from build123d import *

# Parameters (mm, degrees)
SKETCH1_R                = 30
SKETCH1_R_2              = 25
BOSS_EXTRUDE1_DEPTH      = 5
SKETCH2_R                = 25
BOSS_EXTRUDE2_DEPTH      = 2
CUT_EXTRUDE1_DEPTH       = 43.720018727
CUT_EXTRUDE1_DEPTH_BACK  = 43.720018727
SKETCH2_4_R              = 5
BOSS_EXTRUDE3_DEPTH      = 3
BOSS_EXTRUDE3_DEPTH_BACK = 7
SKETCH3_R                = 5
SKETCH3_R_2              = 2
CUT_EXTRUDE2_DEPTH       = 44
CUT_EXTRUDE2_DEPTH_BACK  = 44
SKETCH4_R                = 5
CHAMFER1_SIZE            = 0.5


with BuildPart() as part:
    # Sketch1 → Boss-Extrude1 (new, symmetric)
    with BuildSketch(Plane.XY):
        Circle(SKETCH1_R)
        Circle(SKETCH1_R_2, mode=Mode.SUBTRACT)
    extrude(amount=BOSS_EXTRUDE1_DEPTH, both=True)

    # Sketch2 → Boss-Extrude2 (add, symmetric)
    with BuildSketch(Plane.XY):
        Circle(SKETCH2_R)
    extrude(amount=BOSS_EXTRUDE2_DEPTH, both=True)

    # Sketch2_4 → Cut-Extrude1 (cut, two sides: drawn at the far end of the back side and taken through both)
    with BuildSketch(Plane.XY.offset(-CUT_EXTRUDE1_DEPTH_BACK)):
        Circle(SKETCH2_4_R)
    extrude(amount=CUT_EXTRUDE1_DEPTH + CUT_EXTRUDE1_DEPTH_BACK, mode=Mode.SUBTRACT)

    # Sketch3 → Boss-Extrude3 (add, two sides: drawn at the far end of the back side and taken through both)
    with BuildSketch(Plane(origin=(0, 0, -2), x_dir=(-1, 0, 0), z_dir=(0, 0, -1)).offset(-BOSS_EXTRUDE3_DEPTH_BACK)):
        Circle(SKETCH3_R)
        Circle(SKETCH3_R_2, mode=Mode.SUBTRACT)
    extrude(amount=BOSS_EXTRUDE3_DEPTH + BOSS_EXTRUDE3_DEPTH_BACK)

    # Sketch4 → Cut-Extrude2 (cut, two sides: drawn at the far end of the back side and taken through both)
    with BuildSketch(Plane(origin=(0, 0, -2), x_dir=(-1, 0, 0), z_dir=(0, 0, -1)).offset(-CUT_EXTRUDE2_DEPTH_BACK)):
        with Locations(Location((0, 18, 0), (0, 0, 180))):
            Circle(SKETCH4_R)
        with Locations(Location((12.727922061, 12.727922061, 0), (0, 0, 180))):
            Circle(SKETCH4_R)
        with Locations(Location((18, 0, 0), (0, 0, 180))):
            Circle(SKETCH4_R)
        with Locations(Location((12.727922061, -12.727922061, 0), (0, 0, 180))):
            Circle(SKETCH4_R)
        with Locations(Location((0, -18, 0), (0, 0, 180))):
            Circle(SKETCH4_R)
        with Locations(Location((-12.727922061, -12.727922061, 0), (0, 0, 180))):
            Circle(SKETCH4_R)
        with Locations(Location((-18, 0, 0), (0, 0, 180))):
            Circle(SKETCH4_R)
        with Locations(Location((-12.727922061, 12.727922061, 0), (0, 0, 180))):
            Circle(SKETCH4_R)
    extrude(amount=CUT_EXTRUDE2_DEPTH + CUT_EXTRUDE2_DEPTH_BACK, mode=Mode.SUBTRACT)

    # Chamfer1
    chamfer1_edges = [part.edges().sort_by_distance(p)[0] for p in [
        (-30, 0, -5),
        (-30, 0, 5),
        (-25, 0, -5),
        (-25, 0, 5),
    ]]
    chamfer(chamfer1_edges, length=CHAMFER1_SIZE)


solid = part.part
The listing builds one solid part. Answer for the finished solid, in the listing's coordinates (mm). A direction names the side the tool comes from. Round coordinates to 2 decimals unless told otherwise and drop trailing zeros. Order: outer loops, then holes, each group sorted by start corner. A loop starts at its lowest first (then second) coordinate and runs counter-clockwise, first axis right, second up. Notation, with made-up numbers: M 31.25,58.5 L 49.25,58.5 A12 ccw 49.25,70.5 Z; hole C -29,66.25 d8. An arc over 180 degrees is marked long. Answer in a Markdown table with one row per item. Add a question column.
1) Which of the six approach directions +Z, -Z, +X, -X, +Y, -Y give full straight-line access (tool end or side, diameter ignored) to faces 4 (the face through (0.1, -2.2, 5)), 5 (the face through (-0.3, -5.2, -2)), 6 (the face through (-0.3, -5.2, 2))?
2) The part is cut by section B-B on z = -0.5. Count the separate pieces of the cut face and the enclosed holes in it, plus the area to 3 significant figures.
3) Determine the mould class of faces 1 (the face through (11.644, -7.847, 0.028)), 2 (the face through (-13.2, 22, -5)), 3 (the face through (-29.97, 1.32, 0.06)) for opening direction X: pulls with the +X half, pulls with the -X half, needs draft (parallel to the pull), parting line crosses it, or undercut.
4) Flat-ended cylindrical pins translate along their axes: pin 1 Ø11.5 at (x, y) = (-18, 0) entering from -Z; pin 2 Ø13 at (x, y) = (12.73, 12.73) entering from +Z; pin 3 Ø4 at (y, z) = (-11, -2.5) entering from +X; pin 4 Ø6.5 at (x, y) = (0, 0) entering from +Z. Find the tip coordinate at first contact, or state that the pin passes through.
5) The part is cut by section A-A on z = -3.5. Determine the outline of the cut face in (x, y), plus the area to 3 significant figures.
6) Consider line 1 along Z through (x, y) = (3, 13); line 2 along Y through (x, z) = (-10.5, 3.5); line 3 along Y through (x, z) = (-11.5, -0.75). Determine where each line is inside the solid, lowest interval first. Write a range as from..to.
Findings below:
| question | item | result |
|---|---|---|
| 1 | face 4 | +Z, +X, -X, +Y, -Y |
| 1 | face 5 | -Z |
| 1 | face 6 | +Z |
| 2 | separate pieces | 1 |
| 2 | enclosed holes | 9 |
| 2 | area | 2,190 mm² |
| 3 | face 1 | undercut |
| 3 | face 2 | needs draft |
| 3 | face 3 | parting line crosses it |
| 4 | pin 1 | stops at z = -2 |
| 4 | pin 2 | stops at z = 2 |
| 4 | pin 3 | stops at x = 28.62 |
| 4 | pin 4 | stops at z = 5 |
| 5 | outline | C 0,0 d60; C 0,0 d10; hole C 0,0 d50; hole C 0,0 d4 |
| 5 | area | 930 mm² |
| 6 | line 1 | z = -2..2 |
| 6 | line 2 | y = -28.1..-22.69, 22.69..28.1 |
| 6 | line 3 | y = -27.71..-17.57, -7.88..7.88, 17.57..27.71 |
